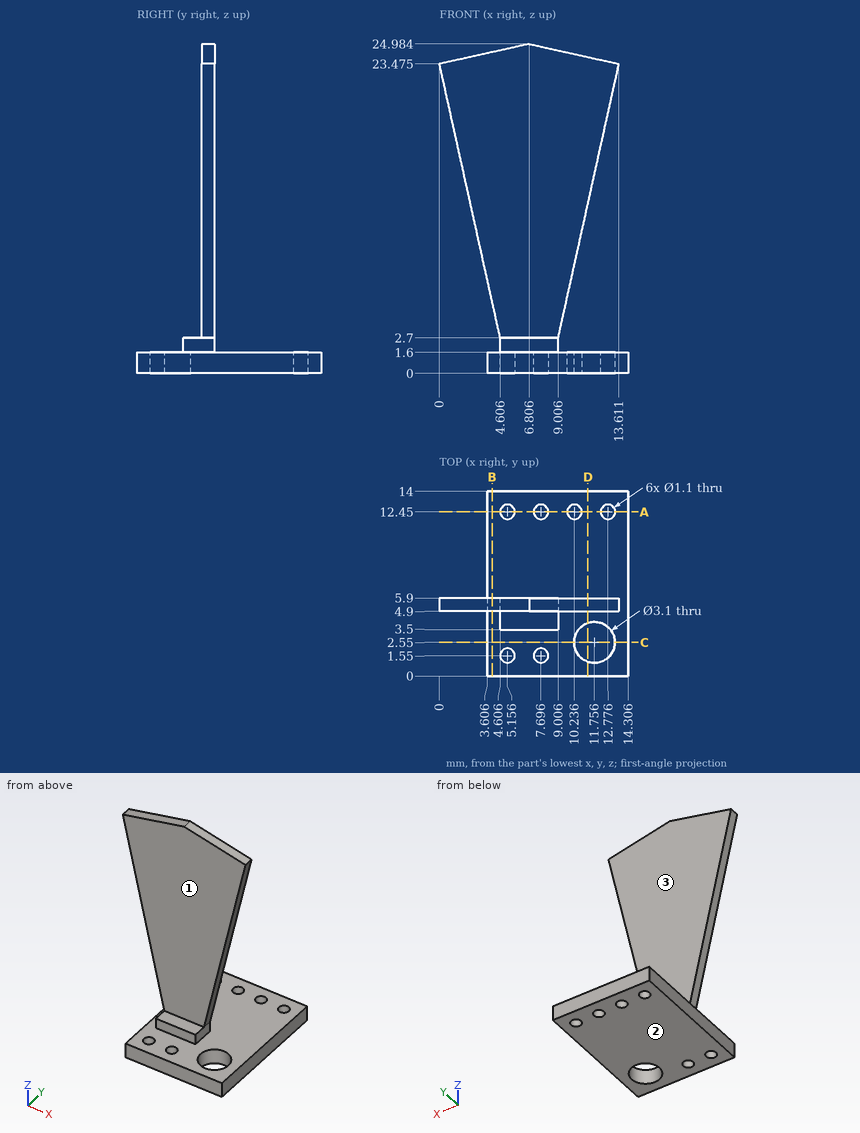
Geometry check sheet. Reference: drawing and pictorial views, mm from the part's lowest x, y, z. A direction names the side the tool comes from. Give positions to 0.01 mm unless a question says otherwise; leave off trailing zeros. Write each loop counter-clockwise with the first axis right and the second up, starting at its lowest first coordinate (ties: lowest second). Pieces come first, ordered by that corner, then holes.
Item 1: Cross-section at C-C (y = 2.55). Enter the section's corners in (x, z) (1 decimal).
Item 2: Cross-section at D-D (x = 11.25). Enter the section's corners in (y, z) (1 decimal).
Item 3: Cross-section at B-B (x = 4). Enter the section's corners in (y, z).
Item 4: Cross-section at A-A (y = 12.45). Enter the section's corners in (x, z) (1 decimal).
Item 5: Access from +Z, -Z, +X, -X, +Y, -Y to the whole of each face (thin tool, end or side, straight path). Record for the marked faces 1, 2 and 3.
Item 6: Scan lines: L1, parallel to Y at x = 7.25, z = 1.5 (1 decimal); L2, parallel to Z at x = 5.5, y = 11.25; L3, parallel to Y at x = 6, z = 10. Record each from-to range of solid material in increasing order.
Item 7: Gauge pin test, flat ends, axial feed: pin 1 (1 mm diameter, centred on x = 8.5, z = 16, fed in from -Y); pin 2 (0.8 mm diameter, centred on y = 7.5, z = 0.5, fed in from -X); pin 3 (1.8 mm diameter, centred on x = 12.78, y = 12.45, fed in from +Z). Record the tip position at first contact, or that the pin passes through.
Report:
1. outline: (3.6, 0) - (10.2, 0) - (10.2, 1.6) - (3.6, 1.6) - close; (13.3, 0) - (14.3, 0) - (14.3, 1.6) - (13.3, 1.6) - close
2. outline: (0, 0) - (1.1, 0) - (1.1, 1.6) - (0, 1.6) - close; (4, 0) - (14, 0) - (14, 1.6) - (4, 1.6) - close; (4.9, 12.8) - (5.9, 12.8) - (5.9, 24) - (4.9, 24) - close
3. outline: (0, 0) - (14, 0) - (14, 1.6) - (0, 1.6) - close; (4.9, 5.43) - (5.9, 5.43) - (5.9, 24.36) - (4.9, 24.36) - close
4. outline: (3.6, 0) - (4.6, 0) - (4.6, 1.6) - (3.6, 1.6) - close; (5.7, 0) - (7.1, 0) - (7.1, 1.6) - (5.7, 1.6) - close; (8.2, 0) - (9.7, 0) - (9.7, 1.6) - (8.2, 1.6) - close; (10.8, 0) - (12.2, 0) - (12.2, 1.6) - (10.8, 1.6) - close; (13.3, 0) - (14.3, 0) - (14.3, 1.6) - (13.3, 1.6) - close
5. face 1: +Z, +X, -X, -Y
5. face 2: -Z, +X, -X, +Y, -Y
5. face 3: +Z, +X, -X, +Y
6. L1: y = 0 to 1.2, 1.9 to 12.1, 12.8 to 14
6. L2: z = 0 to 1.6
6. L3: y = 4.9 to 5.9
7. pin 1: stops at y = 4.9
7. pin 2: stops at x = 3.61
7. pin 3: stops at z = 1.6
